Verification items for the finished model (mm, model axes). Face numbers are marked on the shaded views. Round coordinates to 2 decimals unless told otherwise and drop trailing zeros. Loops run counter-clockwise (first coordinate to the right, second up) from the corner with the lowest first, then second, coordinate; pieces in that order, holes last. Notation, with made-up numbers: (-23.5, 82.25) - (6.5, 82.25) arc R17 ccw to (6.5, 91.25) - close; hole circle Ø5 at (38, -38.5). An arc over 180 degrees is marked (long way). Use a Markdown table: item, result. Add a question column.
```python
from build123d import *

# Parameters (mm, degrees)
F0_W     = 254
F0_H     = 254
F1_DEPTH = 25
F2_R     = 80.732705
F3_DEPTH = 10
F4_R     = 24.252293
F5_DEPTH = 1270
F6_R     = 10.145806
F7_DEPTH = 5


with BuildPart() as f1:
    # F0 (on Top) → F1 (new body)
    with BuildSketch(Plane.XY):
        Rectangle(F0_W, F0_H)
    extrude(amount=F1_DEPTH)

    # F2 (on face) → F3 (join)
    with BuildSketch(Plane.XY.offset(25)):
        Circle(F2_R)
    extrude(amount=F3_DEPTH)

    # F4 (on face) → F5 (cut)
    with BuildSketch(Plane.XY.offset(35)):
        Circle(F4_R)
    extrude(amount=-F5_DEPTH, mode=Mode.SUBTRACT)

    # F6 (on face) → F7 (cut)
    with BuildSketch(Plane.XY.offset(35)):
        with Locations((-51.386729, -42.582173)):
            Circle(F6_R)
    extrude(amount=-F7_DEPTH, mode=Mode.SUBTRACT)


solid = f1.part
```
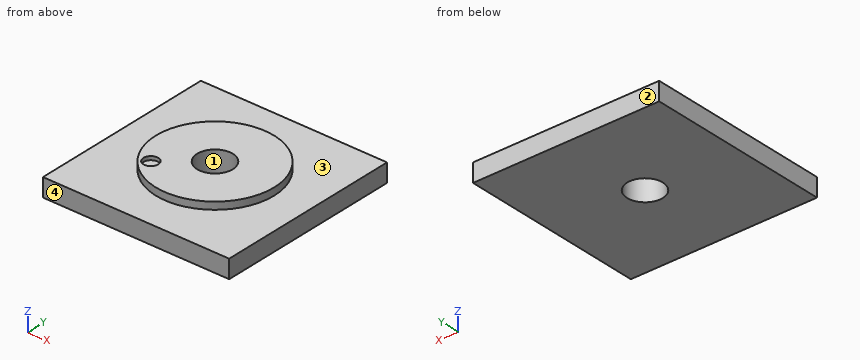
Q1. Thickness scan on line 1 along Y through (x, z) = (0, 28); line 2 along Y through (x, z) = (0, 13); line 3 along Z through (x, y) = (-12, 111.5). Record the ranges inside material, lowest first.
Q2. Section check C-C on z = 17. Record the cut outline in (x, y).
Q3. Section check D-D on x = -69. Record the cut outline in (y, z).
Q4. Release check for a two-part mould opening along Y. For the marked faces 1, 2, 3 and 4 record: +Y half, -Y half, draft (parallel to the pull), parting line (faces both ways), or undercut.
Q5. Go/stop test with flat-tipped pins: pin 1 Ø2 at (y, z) = (-13, 28.5) entering from +X; pin 2 Ø10 at (x, y) = (-51, -44.5) entering from +Z; pin 3 Ø1 at (y, z) = (17, 26) entering from +X. Record where each tip stops, or that it passes through.
Q6. Section check A-A on x = 0. Record the cut outline in (y, z), plus the area to 3 significant figures.
Determined:
| question | item | result |
|---|---|---|
| 1 | line 1 | y = -80.73 to -24.25, 24.25 to 80.73 |
| 1 | line 2 | y = -127 to -24.25, 24.25 to 127 |
| 1 | line 3 | z = 0 to 25 |
| 2 | outline | (-127, -127) - (127, -127) - (127, 127) - (-127, 127) - close; hole circle Ø48.5 at (0, 0) |
| 3 | outline | (-127, 0) - (127, 0) - (127, 25) - (41.91, 25) - (41.91, 35) - (-41.91, 35) - (-41.91, 25) - (-127, 25) - close |
| 4 | face 1 | undercut |
| 4 | face 2 | +Y half |
| 4 | face 3 | draft |
| 4 | face 4 | -Y half |
| 5 | pin 1 | stops at x = 79.84 |
| 5 | pin 2 | stops at z = 30 |
| 5 | pin 3 | stops at x = 79.03 |
| 6 | outline | (-127, 0) - (-24.25, 0) - (-24.25, 35) - (-80.73, 35) - (-80.73, 25) - (-127, 25) - close; (24.25, 0) - (127, 0) - (127, 25) - (80.73, 25) - (80.73, 35) - (24.25, 35) - close |
| 6 | area | 6,270 mm² |
